Build history of the part. All positions in model axes, mm. A direction names the side the tool comes from. Round coordinates to 2 decimals unless told otherwise and drop trailing zeros. Write each loop counter-clockwise with the first axis right and the second up, starting at its lowest first coordinate (ties: lowest second). Pieces come first, ordered by that corner, then holes.
from build123d import *

# Parameters (mm, degrees)
F0_R     = 7.5
F1_DEPTH = 15
F2_R     = 16
F3_DEPTH = 5
F4_R     = 1
F5_SIZE  = 2


with BuildPart() as f1:
    # F0 (on Top) → F1 (new body)
    with BuildSketch(Plane.XY):
        Circle(F0_R)
    extrude(amount=F1_DEPTH)

    # F2 (on face) → F3 (join)
    with BuildSketch(Plane.XY.offset(15)):
        Circle(F2_R)
    extrude(amount=F3_DEPTH)

    # F4
    f4_edges = [f1.edges().sort_by_distance(p)[0] for p in [
        (-16, 0, 20),
        (-16, 0, 15),
    ]]
    fillet(f4_edges, radius=F4_R)

    # F5
    f5_edges = [f1.edges().sort_by_distance(p)[0] for p in [
        (-7.5, 0, 0),
    ]]
    chamfer(f5_edges, length=F5_SIZE)


solid = f1.part
1) Which spindle directions (+Z, -Z, +X, -X, +Y, -Y) get a long thin tool onto all of the face, cutting with end or side? Do faces 1 (the flat face through (0, 0, 20)), 2 (the flat face through (-4, 7, 15)). Say none if no direction does.
Results:
face 1: +Z, +X, -X, +Y, -Y
face 2: -Z
2) Slice it at A-A (x = 0). Write the cut outline in (y, z).
Results:
outline: (-16, 16) arc R1 ccw to (-15, 15) - (-7.5, 15) - (-7.5, 2) - (-5.5, 0) - (5.5, 0) - (7.5, 2) - (7.5, 15) - (15, 15) arc R1 ccw to (16, 16) - (16, 19) arc R1 ccw to (15, 20) - (-15, 20) arc R1 ccw to (-16, 19) - close
3) Wall check: L1, parallel to Z at x = 0, y = 13; L2, parallel to Y at x = 0, z = 11.5; L3, parallel to X at y = 6.5, z = 8.5. Give the ranges that are in metal, low to high.
Results:
L1: z = 15 to 20
L2: y = -7.5 to 7.5
L3: x = -3.74 to 3.74
4) Pin check, flat tips, straight feed: pin 1 Ø6 at (x, z) = (-9, 2.5) entering from -Y; pin 2 Ø15 at (x, y) = (-3.5, -3.5) entering from -Z; pin 3 Ø4 at (x, z) = (-4, 11.5) entering from +Y; pin 4 Ø2 at (x, z) = (4.5, 12) entering from +Y. Stop position of each tip, or through.
Results:
pin 1: stops at y = -4.5
pin 2: stops at z = 0
pin 3: stops at y = 7.23
pin 4: stops at y = 6.63
5) Slice it at D-D (z = 9). Write the cut outline in (x, y).
Results:
outline: circle Ø15 at (0, 0)
6) Slice it at C-C (z = 16.5). Write the cut outline in (x, y).
Results:
outline: circle Ø32 at (0, 0)
